Geometry: see drawing. Coordinates: mm, zero at the bounding-box minimum. A direction names the side the tool comes from. Give positions to 0.01 mm unless a question says otherwise; leave off trailing zeros. Write each loop counter-clockwise with the first axis right and the second up, starting at its lowest first coordinate (ties: lowest second). Pieces come first, ordered by that corner, then holes. Notation, with made-up numbers: (39.25, -3.5) -> (50.25, -3.5) arc R37 ccw to (50.25, 32.5) -> close; hole circle Ø2 at (-10.75, 6.5). An arc over 180 degrees is marked (long way). Answer as a JSON object with one key per item and string values. Group by question number.
Item 1: Section query D-D on x = 14.5. Return the cut outline in (y, z), plus the area to 3 significant figures.
Item 2: Pull-direction query (X, two-part tool) for the marked faces 3, 4, 5 and 6; classes: pulls with the +X half, pulls with the -X half, needs draft (parallel to the pull), parting line crosses it, or undercut.
Item 3: Section query B-B on y = 7. Return the cut outline in (x, z).
Item 4: First-contact query: pin 1 Ø4 at (x, z) = (34.5, 9.5) entering from -Y; pin 2 Ø1.6 at (x, y) = (6.5, 16.5) entering from -Z; pin 3 Ø1 at (y, z) = (34, 3) entering from -X; pin 4 Ø5 at (x, y) = (22, 24.5) entering from -Z. Flat tips, straight axial feed; report the tip coordinate or a pass-through.
Item 5: Section query A-A on z = 17. Return the cut outline in (x, y), plus the area to 3 significant figures.
Item 6: Ray query, probe 1 along X at (y, z) = (32.5, 7); probe 2 along Y at (x, z) = (35, 14.25); probe 3 along Z at (x, y) = (7.5, 12.5). Return the intervals inside material, ascending. Write a range as from..to.
Item 7: Access query for the marked faces 1 and 2. Directions: +Z, -Z, +X, -X, +Y, -Y. A direction counts if a zero-diameter tool reaches every point of the face in a straight line with its end or side. Return the directions, or none.
Item 8: Section query C-C on z = 2. Return the cut outline in (x, y), plus the area to 3 significant figures.
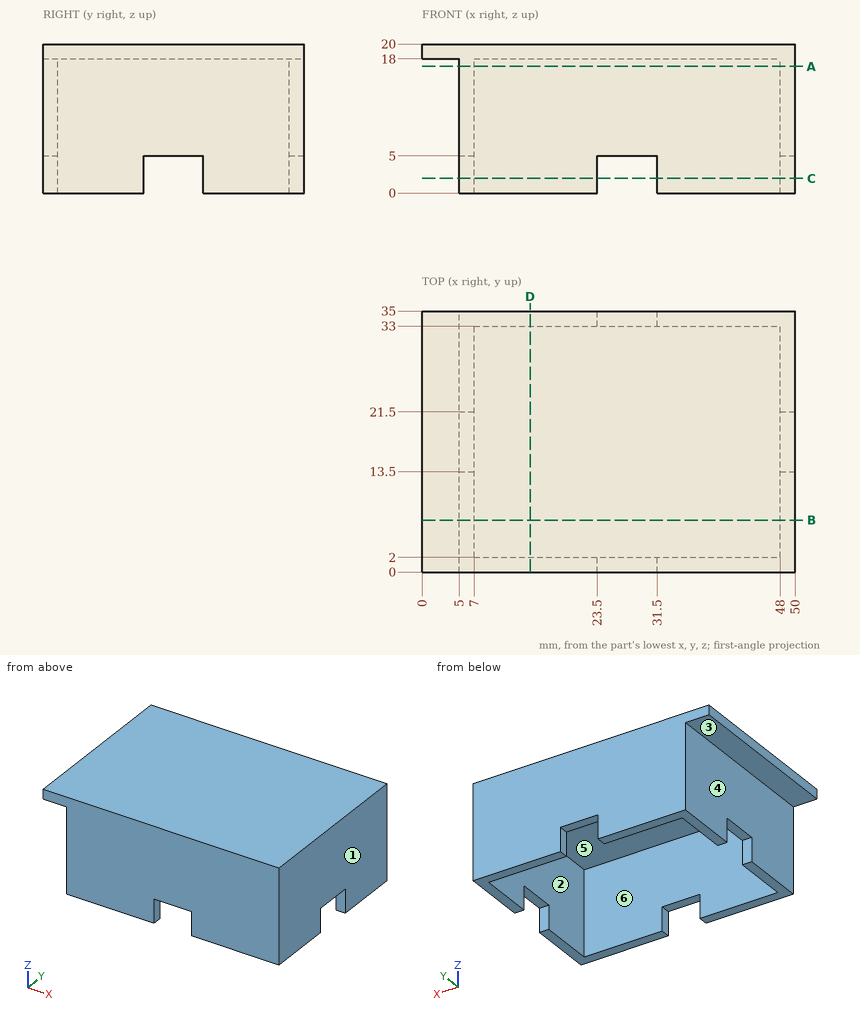
Worked answers:
{
 "1": {"outline": "(0, 0) -> (2, 0) -> (2, 18) -> (33, 18) -> (33, 0) -> (35, 0) -> (35, 20) -> (0, 20) -> close", "area": "142 mm^2"},
 "2": {"face 3": "needs draft", "face 4": "pulls with the -X half", "face 5": "undercut", "face 6": "undercut"},
 "3": {"outline": "(0, 18) -> (5, 18) -> (5, 0) -> (7, 0) -> (7, 18) -> (48, 18) -> (48, 0) -> (50, 0) -> (50, 20) -> (0, 20) -> close"},
 "4": {"pin 1": "y = 0", "pin 2": "z = 5", "pin 3": "x = 5", "pin 4": "z = 18"},
 "5": {"outline": "(5, 0) -> (50, 0) -> (50, 35) -> (5, 35) -> close; hole (7, 2) -> (48, 2) -> (48, 33) -> (7, 33) -> close", "area": "304 mm^2"},
 "6": {"probe 1": "5..7, 48..50", "probe 2": "0..2, 33..35", "probe 3": "18..20"},
 "7": {"face 1": "+Z, -Z, +X, +Y, -Y", "face 2": "-Z"},
 "8": {"outline": "(5, 0) -> (23.5, 0) -> (23.5, 2) -> (7, 2) -> (7, 13.5) -> (5, 13.5) -> close; (5, 21.5) -> (7, 21.5) -> (7, 33) -> (23.5, 33) -> (23.5, 35) -> (5, 35) -> close; (31.5, 0) -> (50, 0) -> (50, 13.5) -> (48, 13.5) -> (48, 2) -> (31.5, 2) -> close; (31.5, 33) -> (48, 33) -> (48, 21.5) -> (50, 21.5) -> (50, 35) -> (31.5, 35) -> close", "area": "240 mm^2"}
}
